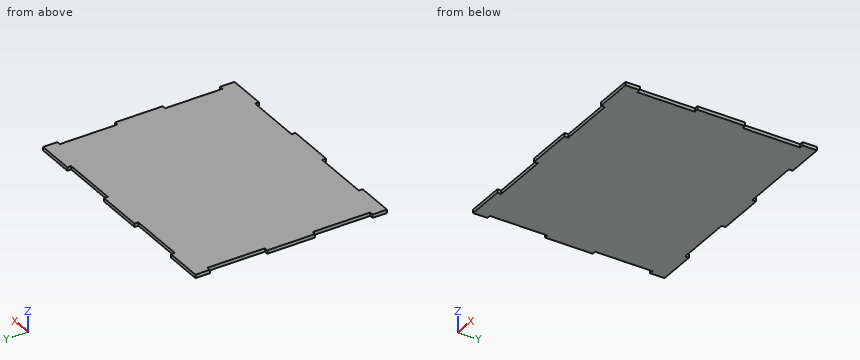
from build123d import *

# Parameters (mm, degrees)
SKETCH_1_W          = 250
SKETCH_1_H          = 200
EXTRUDE_1_DEPTH     = 3.6
SKETCH_2_W          = 4
SKETCH_2_H          = 60
CUT_EXTRUDE_1_DEPTH = 10
SKETCH_3_W          = 60
SKETCH_3_H          = 4
CUT_EXTRUDE_2_DEPTH = 10


with BuildPart() as part:
    # 草图1 → 凸台-拉伸1 (new body)
    with BuildSketch(Plane.XY):
        Rectangle(SKETCH_1_W, SKETCH_1_H)
    extrude(amount=EXTRUDE_1_DEPTH)

    # 草图2 → 切除-拉伸1 (cut)
    with BuildSketch(Plane.XY.offset(3.6)):
        with Locations((-123, 55)):
            Rectangle(SKETCH_2_W, SKETCH_2_H)
        with Locations((123, 55)):
            Rectangle(SKETCH_2_W, SKETCH_2_H)
        with Locations((-123, -55)):
            Rectangle(SKETCH_2_W, SKETCH_2_H)
        with Locations((123, -55)):
            Rectangle(SKETCH_2_W, SKETCH_2_H)
    extrude(amount=-CUT_EXTRUDE_1_DEPTH, mode=Mode.SUBTRACT)

    # 草图3 → 切除-拉伸2 (cut)
    with BuildSketch(Plane.XY.offset(3.6)):
        with Locations((-55, -98)):
            Rectangle(SKETCH_3_W, SKETCH_3_H)
        with Locations((55, -98)):
            Rectangle(SKETCH_3_W, SKETCH_3_H)
        with Locations((55, 98)):
            Rectangle(SKETCH_3_W, SKETCH_3_H)
        with Locations((-55, 98)):
            Rectangle(SKETCH_3_W, SKETCH_3_H)
    extrude(amount=-CUT_EXTRUDE_2_DEPTH, mode=Mode.SUBTRACT)


solid = part.part
Read the model definition and answer for the solid it produces. Units are mm, in the model's axes. Round coordinates to 2 decimals unless told otherwise and drop trailing zeros. Write each loop counter-clockwise with the first axis right and the second up, starting at its lowest first coordinate (ties: lowest second). Pieces come first, ordered by that corner, then holes.
1. The part is cut by section A-A, the plane x = 59. Determine the outline of the cut face in (y, z).
2. Straight lines are drawn through the part: L1, parallel to X at y = 73, z = 1.2; L2, parallel to Y at x = 32.5, z = 1.3. For each, find the intervals that lie inside material, in ascending order.
3. Given pin 1 Ø1.8 at (y, z) = (46, 2.5) entering from -X; pin 2 Ø1.1 at (x, z) = (-50, 2) entering from -Y; pin 3 Ø1.8 at (x, z) = (45.5, 1.5) entering from +Y, each flat-ended and moving along its own axis, determine where each tip first touches the part or whether it passes through.
4. The part is cut by section B-B, the plane y = -36.5. Determine the outline of the cut face in (x, z).
Values:
1. outline: (-96, 0) - (96, 0) - (96, 3.6) - (-96, 3.6) - close
2. L1: x = -121 to 121
2. L2: y = -96 to 96
3. pin 1: stops at x = -121
3. pin 2: stops at y = -96
3. pin 3: stops at y = 96
4. outline: (-121, 0) - (121, 0) - (121, 3.6) - (-121, 3.6) - close
